Source: CAD feature listing. Evaluate the final solid. Frame: model axes, mm. Face numbers are marked on the shaded views. A direction names the side the tool comes from. Give positions to 0.01 mm unless a question says otherwise; leave off trailing zeros. Order: outer loops, then holes, each group sorted by start corner. A loop starts at its lowest first (then second) coordinate and runs counter-clockwise, first axis right, second up.
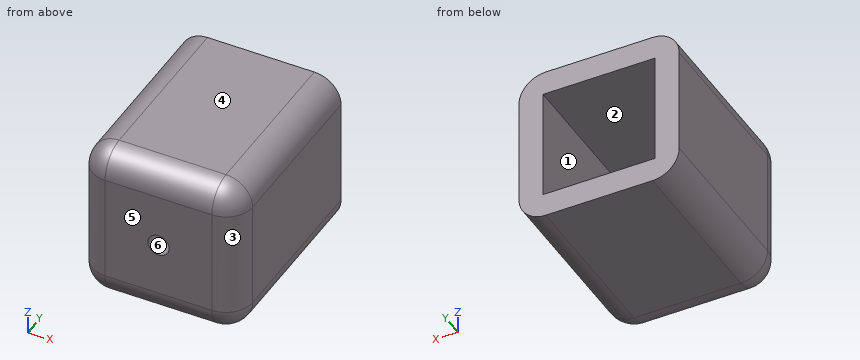
Autodesk Inventor part; units mm, degrees
ref_plane "YZ Plane" through (0, 0, 0) normal (1, 0, 0) x (0, 1, 0)
ref_plane "XZ Plane" through (0, 0, 0) normal (0, 1, 0) x (-1, 0, 0)
ref_plane "XY Plane" through (0, 0, 0) normal (0, 0, 1) x (1, 0, 0)
sketch "Sketch1" plane through (0, 0, 0) normal (0, 1, 0) x (-1, 0, 0)
  line L0 (0, 0) -> (30, 0)
  line L1 (30, 0) -> (30, -30)
  line L2 (30, -30) -> (0, -30)
  line L3 (0, -30) -> (0, 0)
  dimension "d0" = 30
  dimension "d1" = 30
extrude "Extrusion1" add sketch "Sketch1" along normal blind 36.35
sketch "Sketch2" plane through (0, 36.35, 0) normal (0, 1, 0) x (1, 0, 0)
  line L0 (0, 0) -> (0, 30)
  line L1 (0, 0) -> (0, 4.5)
  line L2 (0, 4.5) -> (-4.5, 4.5)
  line L3 (-4.5, 4.5) -> (-25.5, 4.5)
  line L4 (-25.5, 4.5) -> (-25.5, 25.5)
  line L5 (-25.5, 25.5) -> (-4.5, 25.5)
  line L6 (-4.5, 25.5) -> (-4.5, 4.5)
  dimension "d4" = 4.5
  dimension "d5" = 4.5
  dimension "d6" = 21
  dimension "d7" = 21
extrude "Extrusion2" cut sketch "Sketch2" against normal blind 30
sketch "Sketch3" plane through (0, 0, 0) normal (0, -1, 0) x (1, 0, 0)
  line L0 (0, 0) -> (-15, 0)
  line L1 (0, 0) -> (-30, 0)
  line L2 (-15, 0) -> (-15, -15)
  circle A0 centre (-15, -15) radius 2
  dimension "d10" = 15
  dimension "d11" = 4
extrude "Extrusion3" cut sketch "Sketch3" against normal blind 5
fillet "Fillet1" radius 5 4 edges at (0, 0, -15) (-15, 0, 0) (-15, 0, -30) (-30, 0, -15)
fillet "Fillet2" radius 5 8 edges at (-1.4645, 1.4645, -28.5355) (0, 20.675, -30) (-1.4645, 1.4645, -1.4645) (0, 20.675, 0) (-28.5355, 1.4645, -28.5355) (-30, 20.675, -30) (-28.5355, 1.4645, -1.4645) (-30, 20.675, 0)
properties part number "_25in_2020_Endcap"
1) Section query D-D on x = -21. Output: boundary loops of the cut face in (y, z).
Checks:
outline: (0, -25) arc R5 ccw to (5, -30) - (36.35, -30) - (36.35, -25.5) - (6.35, -25.5) - (6.35, -4.5) - (36.35, -4.5) - (36.35, 0) - (5, 0) arc R5 ccw to (0, -5) - close
2) Section query A-A on y = 18.5. Output: boundary loops of the cut face in (x, z), and give its area (3 significant figures).
Checks:
outline: (-30, -25) arc R5 ccw to (-25, -30) - (-5, -30) arc R5 ccw to (0, -25) - (0, -5) arc R5 ccw to (-5, 0) - (-25, 0) arc R5 ccw to (-30, -5) - close; hole (-25.5, -25.5) - (-4.5, -25.5) - (-4.5, -4.5) - (-25.5, -4.5) - close
area: 438 mm2
3) Ray query, L1, parallel to X at y = 22.5, z = -22.25; L2, parallel to Y at x = -12.75, z = -5.25. Return the intervals inside material, ascending.
Checks:
L1: x = -30 to -25.5, -4.5 to 0
L2: y = 0 to 6.35
4) Reachability of the marked faces 5 and 6 from +Z, -Z, +X, -X, +Y, -Y: full face, straight path, thin tool, end or side. Return the list, or none.
Checks:
face 5: +Z, -Z, +X, -X, -Y
face 6: -Y
5) Section query B-B on x = -15. Output: boundary loops of the cut face in (y, z).
Checks:
outline: (0, -25) arc R5 ccw to (5, -30) - (36.35, -30) - (36.35, -25.5) - (6.35, -25.5) - (6.35, -4.5) - (36.35, -4.5) - (36.35, 0) - (5, 0) arc R5 ccw to (0, -5) - (0, -13) - (5, -13) - (5, -17) - (0, -17) - close
6) Section query C-C on z = -23. Output: boundary loops of the cut face in (x, y), and give its area (3 significant figures).
Checks:
outline: (-30, 5) arc R5 ccw to (-25, 0) - (-5, 0) arc R5 ccw to (0, 5) - (0, 36.35) - (-4.5, 36.35) - (-4.5, 6.35) - (-25.5, 6.35) - (-25.5, 36.35) - (-30, 36.35) - close
area: 450 mm2
7) Pull-direction query (Z, two-part tool) for the marked faces 1, 2, 3 and 4; classes: +Z half, -Z half, draft (parallel to the pull), parting line (faces both ways), or undercut.
Checks:
face 1: undercut
face 2: undercut
face 3: draft
face 4: +Z half
